```python
from build123d import *

# Parameters (mm, degrees)
SKETCH_1_R          = 12
EXTRUDE_1_DEPTH     = 9
SKETCH_2_R          = 2
CUT_EXTRUDE_1_DEPTH = 20.209372712
SKETCH_3_R          = 1
CUT_EXTRUDE_2_DEPTH = 3
SKETCH_4_R          = 1.25
CUT_EXTRUDE_3_DEPTH = 13
SKETCH_5_R          = 7.5
SKETCH_5_R_2        = 3.5
CUT_EXTRUDE_4_DEPTH = 0.3


with BuildPart() as part:
    # 草图1 → 凸台-拉伸1 (new body)
    with BuildSketch(Plane(origin=(0, 0, 0), x_dir=(1, 0, 0), z_dir=(0, 1, 0))):
        with Locations(Location((0, 0, 0), (0, 0, 270))):
            Circle(SKETCH_1_R)
    extrude(amount=EXTRUDE_1_DEPTH)

    # 草图2 → 切除-拉伸1 (cut, through all)
    with BuildSketch(Plane(origin=(0, 9, 0), x_dir=(1, 0, 0), z_dir=(0, 1, 0))):
        with Locations(Location((0, 0, 0), (0, 0, 270))):
            Circle(SKETCH_2_R)
    extrude(amount=-CUT_EXTRUDE_1_DEPTH, mode=Mode.SUBTRACT)

    # 草图3 → 切除-拉伸2 (cut)
    with BuildSketch(Plane(origin=(0, 9, 0), x_dir=(1, 0, 0), z_dir=(0, 1, 0))):
        with Locations(Location((0, 9, 0), (0, 0, 270))):
            Circle(SKETCH_3_R)
    extrude(amount=-CUT_EXTRUDE_2_DEPTH, mode=Mode.SUBTRACT)

    # 草图4 → 切除-拉伸3 (cut)
    with BuildSketch(Plane(origin=(0, 0, 0), x_dir=(0, 0, -1), z_dir=(1, 0, 0))):
        with Locations(Location((0, 2.5, 0), (0, 0, 180))):
            Circle(SKETCH_4_R)
    extrude(amount=CUT_EXTRUDE_3_DEPTH, mode=Mode.SUBTRACT)

    # 草图5 → 切除-拉伸4 (cut)
    with BuildSketch(Plane.XZ):
        with Locations(Location((0, 0, 0), (0, 0, 270))):
            Circle(SKETCH_5_R)
        with Locations(Location((0, 0, 0), (0, 0, 270))):
            Circle(SKETCH_5_R_2, mode=Mode.SUBTRACT)
    extrude(amount=-CUT_EXTRUDE_4_DEPTH, mode=Mode.SUBTRACT)


solid = part.part
```
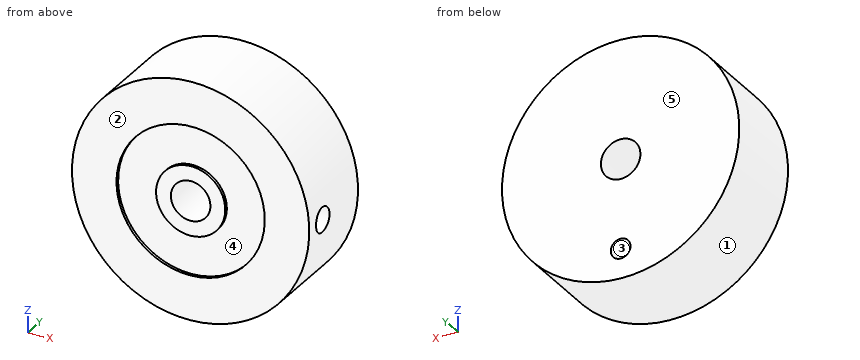
Source: CAD feature listing. Evaluate the final solid. Frame: model axes, mm. Face numbers are marked on the shaded views. A direction names the side the tool comes from. Coordinates: 2 decimals unless noted, no trailing zeros. Write each loop counter-clockwise with the first axis right and the second up, starting at its lowest first coordinate (ties: lowest second). Pieces come first, ordered by that corner, then holes. Notation, with made-up numbers: (29, 62.5) - (87, 62.5) arc R21 cw to (87, 90.5) - close; hole circle Ø11 at (-4, 59.25). An arc over 180 degrees is marked (long way). Answer as a JSON object with one key per item and string values.
Q1. Section query A-A, the plane z = 0. Output: boundary loops of the cut face in (x, y).
Ans:
{"outline": "(-12, 0) - (-7.5, 0) - (-7.5, 0.3) - (-3.5, 0.3) - (-3.5, 0) - (-2, 0) - (-2, 9) - (-12, 9) - close; (2, 0) - (3.5, 0) - (3.5, 0.3) - (7.5, 0.3) - (7.5, 0) - (12, 0) - (12, 1.25) - (2, 1.25) - close; (2, 3.75) - (12, 3.75) - (12, 9) - (2, 9) - close"}
Q2. Set-up query: the marked faces 4 and 5. Return all of +Z, -Z, +X, -X, +Y, -Y with unobstructed straight access to the full face (end or side cutting, diameter ignored); none if empty.
Ans:
{"face 4": "-Y", "face 5": "+Z, -Z, +X, -X, +Y"}
Q3. First-contact query: pin 1 Ø5 at (y, z) = (7, 3) entering from +X; pin 2 Ø1.5 at (x, y) = (2, 2.5) entering from +Z; pin 3 Ø1 at (y, z) = (2.5, -8.5) entering from -X. Flat tips, straight axial feed; report the tip coordinate or a pass-through.
Ans:
{"pin 1": "stops at x = 11.99", "pin 2": "stops at z = 11.93", "pin 3": "stops at x = -8.94"}
Q4. Draft query along X for the marked faces 1, 2 and 3. Return one class per face: released by +X, released by -X, zero draft, split by the parting line, or undercut.
Ans:
{"face 1": "split by the parting line", "face 2": "zero draft", "face 3": "undercut"}
Q5. Section query C-C, the plane y = 7.75. Output: boundary loops of the cut face in (x, z), plus the area to 3 significant figures.
Ans:
{"outline": "circle Ø24 at (0, 0); hole circle Ø4 at (0, 0); hole circle Ø2 at (0, -9)", "area": "437 mm2"}
Q6. Material intervals for line 1 (X direction, y = 4.75, z = 0); line 2 (Y direction, x = 6, z = 0); line 3 (Y direction, x = -0.5, z = -8.75), sorted ascending. Write a range as [from, to].
Ans:
{"line 1": "x = [-12, -2], [2, 12]", "line 2": "y = [0.3, 1.25], [3.75, 9]", "line 3": "y = [0, 6]"}
Q7. Section query B-B, the plane x = 0.5. Output: boundary loops of the cut face in (y, z).
Ans:
{"outline": "(0, -11.99) - (9, -11.99) - (9, -9.87) - (6, -9.87) - (6, -8.13) - (9, -8.13) - (9, -1.94) - (0, -1.94) - (0, -3.46) - (0.3, -3.46) - (0.3, -7.48) - (0, -7.48) - close; (0, 1.94) - (9, 1.94) - (9, 11.99) - (0, 11.99) - (0, 7.48) - (0.3, 7.48) - (0.3, 3.46) - (0, 3.46) - close"}
Q8. Section query D-D, the plane x = 8.75. Output: boundary loops of the cut face in (y, z), plus the area to 3 significant figures.
Ans:
{"outline": "(0, -8.21) - (9, -8.21) - (9, 8.21) - (0, 8.21) - close; hole circle Ø2.5 at (2.5, 0)", "area": "143 mm2"}
